Build history of the part. All positions in model axes, mm. Give positions to 0.01 mm unless a question says otherwise; leave off trailing zeros. Order: outer loops, then holes, each group sorted by start corner. A loop starts at its lowest first (then second) coordinate and runs counter-clockwise, first axis right, second up. Notation, with made-up numbers: (-18.5, 54) - (15.5, 54) arc R32 ccw to (15.5, 92) - close; hole circle Ø11 at (19.25, -6). An arc over 180 degrees is marked (long way). One line per item, written item: value.
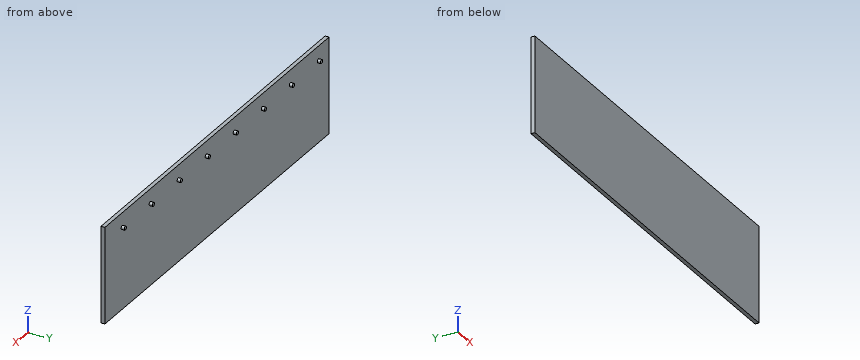
```python
from build123d import *

# Parameters (mm, degrees)
SKETCH1_W           = 159.592906802
SKETCH1_H           = 38.1
BOSS_EXTRUDE1_DEPTH = 1.5875
SKETCH2_R           = 0.75
BOSS_EXTRUDE2_DEPTH = 1.2446
LPATTERN1_COUNT     = 8
LPATTERN1_PITCH     = 19.94911335


with BuildPart() as part:
    # Sketch1 → Boss-Extrude1 (new body)
    with BuildSketch(Plane(origin=(0, 0, 0), x_dir=(1, 0, 0), z_dir=(0, 1, 0))):
        with Locations((79.796453401, 19.05)):
            Rectangle(SKETCH1_W, SKETCH1_H)
    extrude(amount=BOSS_EXTRUDE1_DEPTH)

    # Sketch2 → Boss-Extrude2 (add)
    with BuildSketch(Plane(origin=(0, 1.5875, 0), x_dir=(1, 0, 0), z_dir=(0, 1, 0))):
        with Locations(Location((7.640640269, 5.771220173, 0), (0, 0, 90))):
            Circle(SKETCH2_R)
    boss_extrude2 = extrude(amount=BOSS_EXTRUDE2_DEPTH)

    # LPattern1: Boss-Extrude2 ×8
    with Locations(*[(i * LPATTERN1_PITCH, 0, 0) for i in range(1, LPATTERN1_COUNT)]):
        add(boss_extrude2)


solid = part.part
```
(1) Slice it at A-A, the plane y = 2.1. Give the cut face in (x, z), and give its area (3 significant figures).
Completed:
outline: circle Ø1.5 at (7.64, -5.77); circle Ø1.5 at (27.59, -5.77); circle Ø1.5 at (47.54, -5.77); circle Ø1.5 at (67.49, -5.77); circle Ø1.5 at (87.44, -5.77); circle Ø1.5 at (107.39, -5.77); circle Ø1.5 at (127.34, -5.77); circle Ø1.5 at (147.28, -5.77)
area: 14.1 mm²
(2) Slice it at B-B, the plane z = -25. Give the cut face in (x, y).
Completed:
outline: (0, 0) - (159.59, 0) - (159.59, 1.59) - (0, 1.59) - close
(3) Slice it at C-C, the plane x = 80.5. Give the cut face in (y, z).
Completed:
outline: (0, -38.1) - (1.59, -38.1) - (1.59, 0) - (0, 0) - close
(4) Pin check, flat tips, straight feed: P1, Ø4, axis at x = 76, z = -34, coming from the -Y side; P2, Ø3, axis at x = 74, z = -8.5, coming from the +Y side; P3, Ø1.5, axis at y = 2.5, z = -28, coming from the +X side. Stop position of each tip, or through.
Completed:
P1: y = 0
P2: y = 1.59
P3: through
(5) Drill centre line: line 1 (Y direction, x = 72.5, z = -7). Where is it in solid material? Low to high.
Completed:
line 1: 0 to 1.59
